The listing builds one solid part. Answer for the finished solid, in the listing's coordinates (mm). A direction names the side the tool comes from. Coordinates: 2 decimals unless noted, no trailing zeros. Order: outer loops, then holes, each group sorted by start corner. A loop starts at its lowest first (then second) coordinate and runs counter-clockwise, first axis right, second up. Notation, with made-up numbers: (66.25, -9) -> (110.25, -9) arc R28 cw to (110.25, 14) -> close; hole circle Ø1 at (-34.75, -7). An arc over 180 degrees is marked (long way). Write item = value, one per line.
from build123d import *

# Parameters (mm, degrees)
SKETCH1_R           = 15
BOSS_EXTRUDE1_DEPTH = 2
SKETCH2_R           = 10
BOSS_EXTRUDE2_DEPTH = 2
SKETCH3_R           = 7.5
BOSS_EXTRUDE3_DEPTH = 4
FILLET1_R           = 2
SKETCH4_R           = 5.471529996
BOSS_EXTRUDE4_DEPTH = 7
FILLET2_R           = 5


with BuildPart() as part:
    # Sketch1 → Boss-Extrude1 (new body)
    with BuildSketch(Plane.XY):
        with Locations((-7.532732603, 13.127432061)):
            Circle(SKETCH1_R)
    extrude(amount=BOSS_EXTRUDE1_DEPTH)

    # Sketch2 → Boss-Extrude2 (add)
    with BuildSketch(Plane.XY.offset(2)):
        with Locations((-7.532732603, 13.127432061)):
            Circle(SKETCH2_R)
    extrude(amount=BOSS_EXTRUDE2_DEPTH)

    # Sketch3 → Boss-Extrude3 (add)
    with BuildSketch(Plane.XY.offset(4)):
        with Locations((-7.532732603, 13.127432061)):
            Circle(SKETCH3_R)
    extrude(amount=BOSS_EXTRUDE3_DEPTH)

    # Fillet1
    fillet1_edges = [part.edges().sort_by_distance(p)[0] for p in [
        (-15.032732603, 13.127432061, 8),
    ]]
    fillet(fillet1_edges, radius=FILLET1_R)

    # Sketch4 → Boss-Extrude4 (add)
    with BuildSketch(Plane.XY.offset(8)):
        with Locations((-7.561660228, 13.153988569)):
            Circle(SKETCH4_R)
    extrude(amount=BOSS_EXTRUDE4_DEPTH)

    # Fillet2
    fillet2_edges = [part.edges().sort_by_distance(p)[0] for p in [
        (-13.033190224, 13.153988569, 15),
    ]]
    fillet(fillet2_edges, radius=FILLET2_R)


solid = part.part
Q1. Section C-C, the plane z = 7.5 is taken. Give the vertices of the cut face in (x, y).
The answers:
outline = circle Ø13.65 at (-7.53, 13.13)
Q2. Each of these flat-tipped pins is pushed along its axis until it touches: pin 1 Ø6 at (x, z) = (-15, 7.5) entering from +Y; pin 2 Ø6 at (x, z) = (-12, 4.5) entering from -Y; pin 3 Ø2 at (x, y) = (-6, 10.5) entering from +Z; pin 4 Ø1 at (x, z) = (-13.5, 12.5) entering from -Y. Where does it stop, or does it pass through?
The answers:
pin_1 = 18.94
pin_2 = -1.61
pin_3 = 14.73
pin_4 = through
Q3. Section B-B, the plane y = 4.75 is taken. Give the vertices of the cut face in (x, z), plus the area to 3 significant figures.
The answers:
outline = (-19.98, 0) -> (4.91, 0) -> (4.91, 2) -> (-2.07, 2) -> (-2.07, 4) -> (-12.99, 4) -> (-12.99, 2) -> (-19.98, 2) -> close
area = 71.6 mm2
Q4. Section A-A, the plane x = -15.75 is taken. Give the vertices of the cut face in (y, z).
The answers:
outline = (0.58, 0) -> (25.68, 0) -> (25.68, 2) -> (18.83, 2) -> (18.83, 4) -> (7.43, 4) -> (7.43, 2) -> (0.58, 2) -> close
Q5. Section D-D, the plane x = 4.5 is taken. Give the vertices of the cut face in (y, z).
The answers:
outline = (4.17, 0) -> (22.08, 0) -> (22.08, 2) -> (4.17, 2) -> close
Q6. A tool of negligible diameter and unlimited length cuts with its end or side. For faces 1 (the face through (-10.784, -1.516, 0.986)), 2 (the face through (2.3, 10, 2)), from which of +Z, -Z, +X, -X, +Y, -Y can it reach the whole face along a straight path? Write none if from no direction.
The answers:
face_1 = +Z, -Z
face_2 = +Z
Q7. Find the intervals of material crossed by line 1 along Z through (x, y) = (-1.5, 0); line 2 along Y through (x, z) = (-15.25, 2.75); line 3 along X through (y, z) = (11.5, 13), in increasing order.
The answers:
line_1 = 0 to 2
line_2 = 6.77 to 19.49
line_3 = -11.72 to -3.41
